```python
from build123d import *

# Parameters (mm, degrees)
SKETCH3_R      = 2.6035
EXTRUDE1_DEPTH = 157.05


with BuildPart() as part:
    # Sketch3 → Extrude1 (new, symmetric)
    with BuildSketch(Plane.XY):
        with BuildLine():
            Line((-1.115277175, 4.5085), (1.115277175, 4.5085))
            ThreePointArc((1.115277175, 4.5085), (2.806584872, 4.844922018), (4.240406305, 5.80297087))
            Line((4.240406305, 5.80297087), (7.148423664, 8.710988229))
            ThreePointArc((7.148423664, 8.710988229), (7.349906316, 9.772227925), (6.436353897, 10.348636575))
            Line((6.436353897, 10.348636575), (4.381960454, 10.276895575))
            ThreePointArc((4.381960454, 10.276895575), (3.239173075, 11.342562046), (4.304839546, 12.485349424))
            Line((4.304839546, 12.485349424), (5.728246175, 12.535055879))
            ThreePointArc((5.728246175, 12.535055879), (6.054756855, 12.230579745), (6.35923299, 12.557090424))
            Line((6.35923299, 12.557090424), (9.782092278, 12.676619304))
            ThreePointArc((9.782092278, 12.676619304), (10.108602958, 12.37214317), (10.413079092, 12.69865385))
            ThreePointArc((10.413079092, 12.69865385), (12.052764565, 12.052764565), (12.69865385, 10.413079092))
            ThreePointArc((12.69865385, 10.413079092), (12.37214317, 10.108602958), (12.676619304, 9.782092278))
            Line((12.676619304, 9.782092278), (12.557090424, 6.35923299))
            ThreePointArc((12.557090424, 6.35923299), (12.230579745, 6.054756855), (12.535055879, 5.728246175))
            Line((12.535055879, 5.728246175), (12.485349424, 4.304839546))
            ThreePointArc((12.485349424, 4.304839546), (11.342562046, 3.239173075), (10.276895575, 4.381960454))
            Line((10.276895575, 4.381960454), (10.348636575, 6.436353897))
            ThreePointArc((10.348636575, 6.436353897), (9.772227925, 7.349906316), (8.710988229, 7.148423664))
            Line((8.710988229, 7.148423664), (5.80297087, 4.240406305))
            ThreePointArc((5.80297087, 4.240406305), (4.844922018, 2.806584872), (4.5085, 1.115277175))
            Line((4.5085, 1.115277175), (4.5085, -1.115277175))
            ThreePointArc((4.5085, -1.115277175), (4.844922018, -2.806584872), (5.80297087, -4.240406305))
            Line((5.80297087, -4.240406305), (8.710988229, -7.148423664))
            ThreePointArc((8.710988229, -7.148423664), (9.772227925, -7.349906316), (10.348636575, -6.436353897))
            Line((10.348636575, -6.436353897), (10.276895575, -4.381960454))
            ThreePointArc((10.276895575, -4.381960454), (11.342562046, -3.239173075), (12.485349424, -4.304839546))
            Line((12.485349424, -4.304839546), (12.535055879, -5.728246175))
            ThreePointArc((12.535055879, -5.728246175), (12.230579745, -6.054756855), (12.557090424, -6.35923299))
            Line((12.557090424, -6.35923299), (12.676619304, -9.782092278))
            ThreePointArc((12.676619304, -9.782092278), (12.37214317, -10.108602958), (12.69865385, -10.413079092))
            ThreePointArc((12.69865385, -10.413079092), (12.052764565, -12.052764565), (10.413079092, -12.69865385))
            ThreePointArc((10.413079092, -12.69865385), (10.108602958, -12.37214317), (9.782092278, -12.676619304))
            Line((9.782092278, -12.676619304), (6.35923299, -12.557090424))
            ThreePointArc((6.35923299, -12.557090424), (6.054756855, -12.230579745), (5.728246175, -12.535055879))
            Line((5.728246175, -12.535055879), (4.304839546, -12.485349424))
            ThreePointArc((4.304839546, -12.485349424), (3.239173075, -11.342562046), (4.381960454, -10.276895575))
            Line((4.381960454, -10.276895575), (6.436353897, -10.348636575))
            ThreePointArc((6.436353897, -10.348636575), (7.349906316, -9.772227925), (7.148423664, -8.710988229))
            Line((7.148423664, -8.710988229), (4.240406305, -5.80297087))
            ThreePointArc((4.240406305, -5.80297087), (2.806584872, -4.844922018), (1.115277175, -4.5085))
            Line((1.115277175, -4.5085), (-1.115277175, -4.5085))
            ThreePointArc((-1.115277175, -4.5085), (-2.806584872, -4.844922018), (-4.240406305, -5.80297087))
            Line((-4.240406305, -5.80297087), (-7.148423664, -8.710988229))
            ThreePointArc((-7.148423664, -8.710988229), (-7.349906316, -9.772227925), (-6.436353897, -10.348636575))
            Line((-6.436353897, -10.348636575), (-4.381960454, -10.276895575))
            ThreePointArc((-4.381960454, -10.276895575), (-3.239173075, -11.342562046), (-4.304839546, -12.485349424))
            Line((-4.304839546, -12.485349424), (-5.728246175, -12.535055879))
            ThreePointArc((-5.728246175, -12.535055879), (-6.054756855, -12.230579745), (-6.35923299, -12.557090424))
            Line((-6.35923299, -12.557090424), (-9.782092278, -12.676619304))
            ThreePointArc((-9.782092278, -12.676619304), (-10.108602958, -12.37214317), (-10.413079092, -12.69865385))
            ThreePointArc((-10.413079092, -12.69865385), (-12.052764565, -12.052764565), (-12.69865385, -10.413079092))
            ThreePointArc((-12.69865385, -10.413079092), (-12.37214317, -10.108602958), (-12.676619304, -9.782092278))
            Line((-12.676619304, -9.782092278), (-12.557090424, -6.35923299))
            ThreePointArc((-12.557090424, -6.35923299), (-12.230579745, -6.054756855), (-12.535055879, -5.728246175))
            Line((-12.535055879, -5.728246175), (-12.485349424, -4.304839546))
            ThreePointArc((-12.485349424, -4.304839546), (-11.342562046, -3.239173075), (-10.276895575, -4.381960454))
            Line((-10.276895575, -4.381960454), (-10.348636575, -6.436353897))
            ThreePointArc((-10.348636575, -6.436353897), (-9.772227925, -7.349906316), (-8.710988229, -7.148423664))
            Line((-8.710988229, -7.148423664), (-5.80297087, -4.240406305))
            ThreePointArc((-5.80297087, -4.240406305), (-4.844922018, -2.806584872), (-4.5085, -1.115277175))
            Line((-4.5085, -1.115277175), (-4.5085, 1.115277175))
            ThreePointArc((-4.5085, 1.115277175), (-4.844922018, 2.806584872), (-5.80297087, 4.240406305))
            Line((-5.80297087, 4.240406305), (-8.710988229, 7.148423664))
            ThreePointArc((-8.710988229, 7.148423664), (-9.772227925, 7.349906316), (-10.348636575, 6.436353897))
            Line((-10.348636575, 6.436353897), (-10.276895575, 4.381960454))
            ThreePointArc((-10.276895575, 4.381960454), (-11.342562046, 3.239173075), (-12.485349424, 4.304839546))
            Line((-12.485349424, 4.304839546), (-12.535055879, 5.728246175))
            ThreePointArc((-12.535055879, 5.728246175), (-12.230579745, 6.054756855), (-12.557090424, 6.35923299))
            Line((-12.557090424, 6.35923299), (-12.676619304, 9.782092278))
            ThreePointArc((-12.676619304, 9.782092278), (-12.37214317, 10.108602958), (-12.69865385, 10.413079092))
            ThreePointArc((-12.69865385, 10.413079092), (-12.052764565, 12.052764565), (-10.413079092, 12.69865385))
            ThreePointArc((-10.413079092, 12.69865385), (-10.108602958, 12.37214317), (-9.782092278, 12.676619304))
            Line((-9.782092278, 12.676619304), (-6.35923299, 12.557090424))
            ThreePointArc((-6.35923299, 12.557090424), (-6.054756855, 12.230579745), (-5.728246175, 12.535055879))
            Line((-5.728246175, 12.535055879), (-4.304839546, 12.485349424))
            ThreePointArc((-4.304839546, 12.485349424), (-3.239173075, 11.342562046), (-4.381960454, 10.276895575))
            Line((-4.381960454, 10.276895575), (-6.436353897, 10.348636575))
            ThreePointArc((-6.436353897, 10.348636575), (-7.349906316, 9.772227925), (-7.148423664, 8.710988229))
            Line((-7.148423664, 8.710988229), (-4.240406305, 5.80297087))
            ThreePointArc((-4.240406305, 5.80297087), (-2.806584872, 4.844922018), (-1.115277175, 4.5085))
        make_face()
        Circle(SKETCH3_R, mode=Mode.SUBTRACT)
    extrude(amount=EXTRUDE1_DEPTH, both=True)


solid = part.part
```
Here's how the part is built. I have some questions about the finished solid (model axes, mm). Coordinates: 2 decimals unless noted, no trailing zeros. Answer as a JSON object with one key per item and string values. Group by question number.
(1) I need wall thicknesses on probe 1 along Y at (x, z) = (-4.25, 10.5); probe 2 along Y at (x, z) = (0, -93.5); probe 3 along X at (y, z) = (3.75, 79). Which ranges of each line are inside material? Lowest first, please.
(2) If we mould it in two halves opening along X, with no side actions, what happens to faces 1 (the face through (2.483, 0.782, -2.199)), 2 (the face through (0, 3, 157.05))? For each: released by +X, released by -X, zero draft, split by the parting line, or undercut.
(3) For pin 1 (10 mm diameter, centred on x = 1, z = -0.5, fed in from -Y); pin 2 (2.5 mm diameter, centred on y = 0, z = 26.5, fed in from +X); pin 3 (6 mm diameter, centred on x = -7, z = -116.5, fed in from -Y); pin 4 (8 mm diameter, centred on x = -2, y = 7.5, fed in from -Z), each with a flat end and sliding along its axis, tell me the tip position at first contact or that it passes through.
Values found:
{
 "1": {"probe 1": "y = -12.48 to -10.28, -5.81 to 5.81, 10.28 to 12.48", "probe 2": "y = -4.51 to -2.6, 2.6 to 4.51", "probe 3": "x = -12.31 to -10.45, -5.38 to 5.38, 10.45 to 12.31"},
 "2": {"face 1": "undercut", "face 2": "zero draft"},
 "3": {"pin 1": "stops at y = -12.54", "pin 2": "stops at x = 4.51", "pin 3": "stops at y = -12.68", "pin 4": "stops at z = -157.05"}
}
